Check sheet for the modelled part. Datum: model origin and axes. Units: mm. Face numbers are marked on the shaded views. Round coordinates to 2 decimals unless told otherwise and drop trailing zeros. Order: outer loops, then holes, each group sorted by start corner. A loop starts at its lowest first (then second) coordinate and runs counter-clockwise, first axis right, second up.
Q1. Scan lines: probe 1 along X at (y, z) = (13.45, 0); probe 2 along Y at (x, z) = (-22, 3); probe 3 along X at (y, z) = (3.75, 1). Record each from-to range of solid material in increasing order.
Q2. Cross-section at C-C on x = 0. Record the cut outline in (y, z).
Q3. Mould release check, pull along X, two halves, no side actions. Record for the marked faces 1 and 2: +X half, -X half, draft (parallel to the pull), parting line (faces both ways), or undercut.
Q4. Cross-section at A-A on x = 22.5. Record the cut outline in (y, z), then the cut area to 3 significant figures.
Q5. Cross-section at B-B on z = 0. Give the number of separate pieces and of enclosed holes in the cut face, then the cut area to 3 significant figures.
Q6. Depth check by flat-ended pin: P1, Ø2, axis at x = 13, y = 4, coming from the -Z side; P2, Ø6, axis at x = 22.5, z = 0, coming from the -Y side; P3, Ø1.5, axis at x = 7, y = 11.5, coming from the -Z side. Enter the tip coordinate at first touch or a pass-through.
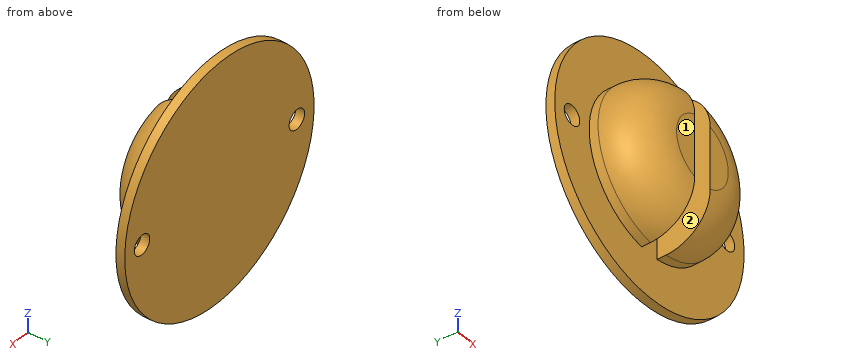
from build123d import *

# Parameters (mm, degrees)
SKETCH1_R           = 17.5
BOSS_EXTRUDE1_DEPTH = 12
SKETCH2_R           = 27.5
BOSS_EXTRUDE2_DEPTH = 2
SKETCH3_W           = 4.5
SKETCH3_H           = 43.807088702
CUT_EXTRUDE2_DEPTH  = 12
FILLET1_R           = 10
SKETCH4_R           = 2.25
CUT_EXTRUDE3_DEPTH  = 101.6


with BuildPart() as part:
    # Sketch1 → Boss-Extrude1 (new body)
    with BuildSketch(Plane(origin=(0, 0, 0), x_dir=(1, 0, 0), z_dir=(0, 1, 0))):
        with Locations(Location((0, 0, 0), (0, 0, 270))):
            Circle(SKETCH1_R)
    extrude(amount=BOSS_EXTRUDE1_DEPTH)

    # Sketch2 → Boss-Extrude2 (add)
    with BuildSketch(Plane(origin=(0, 12, 0), x_dir=(1, 0, 0), z_dir=(0, 1, 0))):
        with Locations(Location((0, 0, 0), (0, 0, 270))):
            Circle(SKETCH2_R)
    extrude(amount=BOSS_EXTRUDE2_DEPTH)

    # Sketch3 → Cut-Extrude2 (cut)
    with BuildSketch(Plane(origin=(0, 0, 0), x_dir=(-1, 0, 0), z_dir=(0, -1, 0))):
        Rectangle(SKETCH3_W, SKETCH3_H)
    extrude(amount=-CUT_EXTRUDE2_DEPTH, mode=Mode.SUBTRACT)

    # Fillet1
    fillet1_edges = [part.edges().sort_by_distance(p)[0] for p in [
        (-17.5, 0, 0),
        (17.5, 0, 0),
    ]]
    fillet(fillet1_edges, radius=FILLET1_R)

    # Sketch4 → Cut-Extrude3 (cut)
    with BuildSketch(Plane(origin=(0, 12, 0), x_dir=(-1, 0, 0), z_dir=(0, -1, 0))):
        with Locations(Location((-22.5, 0, 0), (0, 0, 90))):
            Circle(SKETCH4_R)
        with Locations(Location((22.5, 0, 0), (0, 0, 90))):
            Circle(SKETCH4_R)
    extrude(amount=-CUT_EXTRUDE3_DEPTH, mode=Mode.SUBTRACT)


solid = part.part
Results found:
1. probe 1: x = -27.5 to -24.75, -20.25 to 20.25, 24.75 to 27.5
1. probe 2: y = 12 to 14
1. probe 3: x = -15.27 to -2.25, 2.25 to 15.27
2. outline: (12, -27.5) - (14, -27.5) - (14, 27.5) - (12, 27.5) - close
3. face 1: draft
3. face 2: undercut
4. outline: (12, -15.81) - (14, -15.81) - (14, -2.25) - (12, -2.25) - close; (12, 2.25) - (14, 2.25) - (14, 15.81) - (12, 15.81) - close
4. area: 54.2 mm2
5. separate pieces: 3
5. enclosed holes: 0
5. area: 415 mm2
6. P1: stops at z = -10.22
6. P2: stops at y = 12
6. P3: stops at z = -26.74
